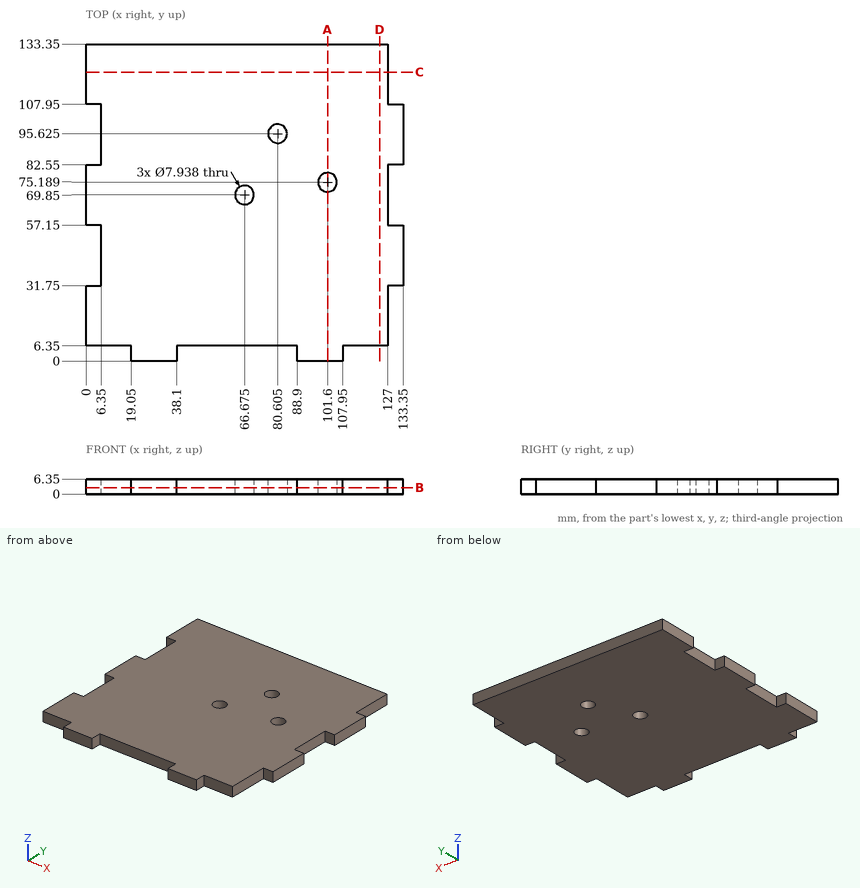
Input: dimensioned drawing with shaded views. Units: mm. Origin: part minimum x, y, z. Coordinates: 2 decimals unless noted, no trailing zeros. Order: outer loops, then holes, each group sorted by start corner. A loop starts at its lowest first (then second) coordinate and runs counter-clockwise, first axis right, second up.
(1) Section query A-A (x = 101.6). Return the cut outline in (y, z).
(2) Section query B-B (z = 2.75). State how many separate pieces and enclosed holes the cut face has, plus the area to 3 significant figures.
(3) First-contact query: pin 1 (1.5 mm diameter, centred on y = 60, z = 2, fed in from +X); pin 2 (3 mm diameter, centred on y = 4, z = 2.5, fed in from +X); pin 3 (1.9 mm diameter, centred on x = 58.5, z = 3, fed in from -Y); pin 4 (12.5 mm diameter, centred on x = 80.61, y = 95.63, fed in from +Z). Flat tips, straight axial feed; report the tip coordinate or a pass-through.
(4) Section query D-D (x = 123.5). Return the cut outline in (y, z).
(5) Section query C-C (y = 121.5). Return the cut outline in (x, z).
(6) Material intervals for probe 1 along Y at (x, z) = (101.6, 4.5); probe 2 along Y at (x, z) = (47.5, 3.75); probe 3 along X at (y, z) = (59, 2.5), sorted ascending.
Solution:
1. outline: (0, 0) - (71.22, 0) - (71.22, 6.35) - (0, 6.35) - close; (79.16, 0) - (133.35, 0) - (133.35, 6.35) - (79.16, 6.35) - close
2. separate pieces: 1
2. enclosed holes: 3
2. area: 16,200 mm2
3. pin 1: stops at x = 127
3. pin 2: stops at x = 107.95
3. pin 3: stops at y = 6.35
3. pin 4: stops at z = 6.35
4. outline: (6.35, 0) - (133.35, 0) - (133.35, 6.35) - (6.35, 6.35) - close
5. outline: (0, 0) - (127, 0) - (127, 6.35) - (0, 6.35) - close
6. probe 1: y = 0 to 71.22, 79.16 to 133.35
6. probe 2: y = 6.35 to 133.35
6. probe 3: x = 0 to 127
